```python
from build123d import *

# Parameters (mm, degrees)
SKETCH1_W           = 20
SKETCH1_H           = 20
BOSS_EXTRUDE1_DEPTH = 10
CUT_EXTRUDE1_DEPTH  = 5
FILLET1_R           = 10


with BuildPart() as part:
    # Sketch1 → Boss-Extrude1 (new body)
    with BuildSketch(Plane(origin=(0, 0, 0), x_dir=(1, 0, 0), z_dir=(0, 1, 0))):
        Rectangle(SKETCH1_W, SKETCH1_H)
    extrude(amount=BOSS_EXTRUDE1_DEPTH)

    # Sketch2 → Cut-Extrude1 (cut)
    with BuildSketch(Plane(origin=(0, 10, 0), x_dir=(1, 0, 0), z_dir=(0, 1, 0))):
        Polygon((0, 3.92598183), (-3.4, 1.962990915), (-3.4, -1.962990915), (0, -3.92598183), (3.4, -1.962990915), (3.4, 1.962990915), align=None)
    extrude(amount=-CUT_EXTRUDE1_DEPTH, mode=Mode.SUBTRACT)

    # Fillet1
    fillet1_edges = [part.edges().sort_by_distance(p)[0] for p in [
        (10, 5, -10),
        (10, 5, 10),
        (-10, 5, -10),
        (-10, 5, 10),
    ]]
    fillet(fillet1_edges, radius=FILLET1_R - 0.0001)  # a hair under: the kernel refuses the full size


solid = part.part
```
Can you work these out from the model? Positions are in its coordinate system, mm. A direction names the side the tool comes from. Give positions to 0.01 mm unless a question says otherwise; leave off trailing zeros. Order: outer loops, then holes, each group sorted by start corner. A loop starts at its lowest first (then second) coordinate and runs counter-clockwise, first axis right, second up. Notation, with made-up numbers: (71, 74.5) - (117, 74.5) arc R29 cw to (117, 107.5) - close; hole circle Ø4 at (26, 37.25). An arc over 180 degrees is marked (long way). Use a Markdown table: item, result. Add a question column.
Q1. I'm going to push flat-ended pins straight in: pin 1 (2 mm diameter, centred on y = 5.5, z = -1.5, fed in from -X); pin 2 (2 mm diameter, centred on y = 7, z = -0.5, fed in from +X); pin 3 (2 mm diameter, centred on x = -1, z = 0.5, fed in from +Y); pin 4 (1.5 mm diameter, centred on x = -4.5, y = 6.5, fed in from -Z). Where does each tip first touch, or does it pass through?
Q2. If we section it at D-D on x = -7.75: Write out the boundary of the cut face in (y, z), plus the area to 3 significant figures.
Q3. On a 3-axis mill with a long thin cutter (end or side, diameter ignored), from which of +Z, -Z, +X, -X, +Y, -Y can I reach the whole of each face in a straight line? I mean faces 4 (the cylindrical face through (-7.15, 5.07, -6.99)), 5 (the flat face through (0, 5, 0)). Say none if no direction works.
Q4. If we mould it in two halves opening along Z, with no side actions, what happens to faces 1 (the flat face through (0, 0, 0)), 2 (the flat face through (-3.4, 8, 0)), 3 (the cylindrical face through (6.99, 5.07, 7.15))? For each: released by +Z, released by -Z, zero draft, split by the parting line, or undercut.
Q5. If we section it at C-C on x = 1: Write out the boundary of the cut face in (y, z), plus the area to 3 significant figures.
Q6. If we section it at B-B on z = 3: Write out the boundary of the cut face in (x, y), plus the area to 3 significant figures.
Q7. Please list where these lines run through material, in increasing order: line 1 along Z through (x, y) = (2.75, 5.25); line 2 along X through (y, z) = (6.75, 0.5); line 3 along Z through (x, y) = (2, 6.25).
Answers follow:
| question | item | result |
|---|---|---|
| 1 | pin 1 | stops at x = -9.99 |
| 1 | pin 2 | stops at x = 10 |
| 1 | pin 3 | stops at y = 5 |
| 1 | pin 4 | stops at z = -9.27 |
| 2 | outline | (0, -6.32) - (10, -6.32) - (10, 6.32) - (0, 6.32) - close |
| 2 | area | 126 mm^2 |
| 3 | face 4 | -Z, -X, +Y, -Y |
| 3 | face 5 | +Y |
| 4 | face 1 | zero draft |
| 4 | face 2 | undercut |
| 4 | face 3 | released by +Z |
| 5 | outline | (0, -9.95) - (10, -9.95) - (10, -3.35) - (5, -3.35) - (5, 3.35) - (10, 3.35) - (10, 9.95) - (0, 9.95) - close |
| 5 | area | 166 mm^2 |
| 6 | outline | (-9.54, 0) - (9.54, 0) - (9.54, 10) - (1.6, 10) - (1.6, 5) - (-1.6, 5) - (-1.6, 10) - (-9.54, 10) - close |
| 6 | area | 175 mm^2 |
| 7 | line 1 | z = -9.61 to -2.34, 2.34 to 9.61 |
| 7 | line 2 | x = -9.99 to -3.4, 3.4 to 9.99 |
| 7 | line 3 | z = -9.8 to -2.77, 2.77 to 9.8 |
